Read the model definition and answer for the solid it produces. Units are mm, in the model's axes. A direction names the side the tool comes from. Round coordinates to 2 decimals unless told otherwise and drop trailing zeros. Loops run counter-clockwise (first coordinate to the right, second up) from the corner with the lowest first, then second, coordinate; pieces in that order, holes last. Notation, with made-up numbers: M -18,-4 L -8,-4 A27 ccw -8,27 Z; hole C 38,44.5 d1. An arc over 180 degrees is marked long. Answer as CSV lines item,"result".
```python
from build123d import *

# Parameters (mm, degrees)
ESBO_O1_W                = 25
ESBO_O1_H                = 15
RESSALTO_EXTRUS_O1_DEPTH = 3
ESBO_O3_W                = 3
ESBO_O3_H                = 15
RESSALTO_EXTRUS_O2_DEPTH = 3
ESBO_O5_W                = 3
ESBO_O5_H                = 15
RESSALTO_EXTRUS_O3_DEPTH = 30
ESBO_O8_W                = 25
ESBO_O8_H                = 15
RESSALTO_EXTRUS_O4_DEPTH = 1
ESBO_O9_R                = 1.75
CORTE_EXTRUS_O1_DEPTH    = 44.720704477
ESBO_O10_W               = 4
ESBO_O10_H               = 15
RESSALTO_EXTRUS_O5_DEPTH = 13
ESBO_O11_R               = 1.75
CORTE_EXTRUS_O2_DEPTH    = 44.341665866


with BuildPart() as part:
    # Esboço1 → Ressalto-extrusão1 (new body)
    with BuildSketch(Plane.XY):
        Rectangle(ESBO_O1_W, ESBO_O1_H)
    extrude(amount=RESSALTO_EXTRUS_O1_DEPTH)

    # Esboço3 → Ressalto-extrusão2 (add)
    with BuildSketch(Plane.XY.offset(3)):
        with Locations((11, 0)):
            Rectangle(ESBO_O3_W, ESBO_O3_H)
    extrude(amount=RESSALTO_EXTRUS_O2_DEPTH)

    # Esboço5 → Ressalto-extrusão3 (add)
    with BuildSketch(Plane(origin=(12.5, 0, 0), x_dir=(0, 0, -1), z_dir=(1, 0, 0))):
        with Locations((-4.5, 0)):
            Rectangle(ESBO_O5_W, ESBO_O5_H)
    extrude(amount=RESSALTO_EXTRUS_O3_DEPTH)

    # Esboço8 → Ressalto-extrusão4 (add)
    with BuildSketch(Plane(origin=(0, 0, 0), x_dir=(-1, 0, 0), z_dir=(0, 0, -1))):
        Rectangle(ESBO_O8_W, ESBO_O8_H)
    extrude(amount=RESSALTO_EXTRUS_O4_DEPTH)

    # Esboço9 → Corte-extrusão1 (cut, through all)
    with BuildSketch(Plane(origin=(0, 0, -1), x_dir=(-1, 0, 0), z_dir=(0, 0, -1))):
        with Locations((-6.5, 0)):
            Circle(ESBO_O9_R)
        with Locations(Location((6.5, 0, 0), (0, 0, 180))):
            Circle(ESBO_O9_R)
    extrude(amount=-CORTE_EXTRUS_O1_DEPTH, mode=Mode.SUBTRACT)

    # Esboço10 → Ressalto-extrusão5 (add)
    with BuildSketch(Plane.ZY.offset(12.5)):
        with Locations((1, 0)):
            Rectangle(ESBO_O10_W, ESBO_O10_H)
    extrude(amount=RESSALTO_EXTRUS_O5_DEPTH)

    # Esboço11 → Corte-extrusão2 (cut, through all)
    with BuildSketch(Plane.XY.offset(3)):
        with Locations((-19.5, 0)):
            Circle(ESBO_O11_R)
    extrude(amount=-CORTE_EXTRUS_O2_DEPTH, mode=Mode.SUBTRACT)


solid = part.part
```
1) A tool of negligible diameter and unlimited length cuts with its end or side. For faces 4 (the cylindrical face through (5.69, -1.55, 0.97)), 5 (the flat face through (-8, -2, 3)), 6 (the flat face through (12.5, 0, 1)), from which of +Z, -Z, +X, -X, +Y, -Y can it reach the whole face along a straight path? Write none if from no direction.
Evaluation:
face 4,"+Z, -Z"
face 5,"+Z, -X, +Y, -Y"
face 6,"-Z, +X, +Y, -Y"
2) Find section A-A, the plane x = 6.5. Give the vertices of the cut face in (y, z), then the cut area to 3 significant figures.
Evaluation:
outline,"M -7.5,-1 L -1.75,-1 L -1.75,3 L -7.5,3 Z; M 1.75,-1 L 7.5,-1 L 7.5,3 L 1.75,3 Z"
area,"46.0 mm^2"
3) Straight lines are drawn through the part: line 1 (Y direction, x = 6.5, z = 0.8); line 2 (X direction, y = 0.75, z = -0.25); line 3 (Z direction, x = -14.5, y = 2.5). For each, find the intervals that lie inside material, in ascending order.
Evaluation:
line 1,"y = -7.5 to -1.75, 1.75 to 7.5"
line 2,"x = -25.5 to -21.08, -17.92 to -8.08, -4.92 to 4.92, 8.08 to 12.5"
line 3,"z = -1 to 3"
4) Each of these flat-tipped pins is pushed along its axis until it touches: P1, Ø3, axis at x = -19.5, y = 0, coming from the -Z side; P2, Ø1.2, axis at y = -2.5, z = 0.5, coming from the +X side; P3, Ø4.5, axis at x = 31.5, y = -1.5, coming from the -Z side; P4, Ø5.5, axis at x = -6.5, y = 0, coming from the -Z side. Where does it stop, or does it pass through?
Evaluation:
P1,"passes through"
P2,"stops at x = 12.5"
P3,"stops at z = 3"
P4,"stops at z = -1"
5) Find section B-B, the plane z = 0.5. Give the vertices of the cut face in (x, y), then the cut area to 3 significant figures.
Evaluation:
outline,"M -25.5,-7.5 L 12.5,-7.5 L 12.5,7.5 L -25.5,7.5 Z; hole C -19.5,0 d3.5; hole C -6.5,0 d3.5; hole C 6.5,0 d3.5"
area,"541 mm^2"
6) Determine the mould class of faces 1 (the flat face through (42.5, 0, 5)), 2 (the flat face through (-25.5, 0, 1)), 3 (the cylindrical face through (-21.25, 0.08, 1.03)) for opening direction X: released by +X, released by -X, zero draft, split by the parting line, or undercut.
Evaluation:
face 1,"released by +X"
face 2,"released by -X"
face 3,"undercut"
7) Find section C-C, the plane y = 4.5. Give the vertices of the cut face in (x, z), then the cut area to 3 significant figures.
Evaluation:
outline,"M -25.5,-1 L 12.5,-1 L 12.5,3 L 42.5,3 L 42.5,6 L 9.5,6 L 9.5,3 L -25.5,3 Z"
area,"251 mm^2"
8) Find section D-D, the plane z = 4. Give the vertices of the cut face in (x, y), then the cut area to 3 significant figures.
Evaluation:
outline,"M 9.5,-7.5 L 42.5,-7.5 L 42.5,7.5 L 9.5,7.5 Z"
area,"495 mm^2"
